Geometry check sheet. Reference: the model listing, model coordinates, mm. A direction names the side the tool comes from. Round coordinates to 2 decimals unless told otherwise and drop trailing zeros. Order: outer loops, then holes, each group sorted by start corner. A loop starts at its lowest first (then second) coordinate and runs counter-clockwise, first axis right, second up. Notation, with made-up numbers: M -6.5,-31 L 47.5,-31 A22 cw 47.5,-4 Z; hole C 79.25,78.5 d3. An arc over 180 degrees is marked long. Answer as a JSON object with one key per item and string values. Group by question number.
```python
from build123d import *

# Parameters (mm, degrees)
BOSS_EXTRUDE1_DEPTH = 2
SKETCH2_R           = 5
BOSS_EXTRUDE3_DEPTH = 4
SKETCH5_R           = 3
CUT_EXTRUDE1_DEPTH  = 4
SKETCH6_R           = 1.5
CUT_EXTRUDE2_DEPTH  = 2
SKETCH7_R           = 2.5
CUT_EXTRUDE4_DEPTH  = 3


with BuildPart() as part:
    # Sketch1 → Boss-Extrude1 (new body)
    with BuildSketch(Plane(origin=(0, 0, 0), x_dir=(1, 0, 0), z_dir=(0, 1, 0))):
        with BuildLine():
            Line((0, 7.598649923), (20, 7.598649923))
            ThreePointArc((20, 7.598649923), (27.5, 0.098649923), (20, -7.401350077))
            Line((20, -7.401350077), (0, -7.401350077))
            ThreePointArc((0, -7.401350077), (-7.5, 0.098649923), (0, 7.598649923))
        make_face()
    extrude(amount=BOSS_EXTRUDE1_DEPTH)

    # Sketch2 → Boss-Extrude3 (add)
    with BuildSketch(Plane(origin=(0, 2, 0), x_dir=(1, 0, 0), z_dir=(0, 1, 0))):
        Circle(SKETCH2_R)
    extrude(amount=BOSS_EXTRUDE3_DEPTH)

    # Sketch5 → Cut-Extrude1 (cut)
    with BuildSketch(Plane(origin=(0, 6, 0), x_dir=(1, 0, 0), z_dir=(0, 1, 0))):
        Circle(SKETCH5_R)
    extrude(amount=-CUT_EXTRUDE1_DEPTH, mode=Mode.SUBTRACT)

    # Sketch6 → Cut-Extrude2 (cut)
    with BuildSketch(Plane(origin=(0, 2, 0), x_dir=(1, 0, 0), z_dir=(0, 1, 0))):
        Circle(SKETCH6_R)
    extrude(amount=-CUT_EXTRUDE2_DEPTH, mode=Mode.SUBTRACT)

    # Sketch7 → Cut-Extrude4 (cut, through all)
    with BuildSketch(Plane(origin=(0, 2, 0), x_dir=(1, 0, 0), z_dir=(0, 1, 0))):
        with Locations((12.2, 0)):
            Circle(SKETCH7_R)
    extrude(amount=-CUT_EXTRUDE4_DEPTH, mode=Mode.SUBTRACT)


solid = part.part
```
1) Sectioned sample at B-B (y = 0.95). Record the boundary of the cut face in (x, z), then the cut area to 3 significant figures.
2) Go/stop test with flat-tipped pins: P1, Ø1.8, axis at x = -1, z = -0.5, coming from the +Y side; P2, Ø1, axis at x = 21, y = 1, coming from the -Z side. Record where each tip stops, or that it passes through.
3) Sectioned sample at D-D (y = 3.75). Record the boundary of the cut face in (x, z), then the cut area to 3 significant figures.
4) Sectioned sample at C-C (z = 1). Record the boundary of the cut face in (x, y), then the cut area to 3 significant figures.
5) Sectioned sample at A-A (x = 12.2). Record the boundary of the cut face in (y, z), then the cut area to 3 significant figures.
6) Thickness scan on line 1 along X through (y, z) = (0.5, 0); line 2 along Z through (x, y) = (12.2, 0.85); line 3 along Y through (x, z) = (24, 1.25). Record the ranges inside material, lowest first. Write a range as [from, to].
7) Release check for a two-part mould opening along X. For faces 1 (the cylindrical face through (-1.08, 3.97, 4.88)), 2 (the cylindrical face through (-3, 4, 0)), 3 (the cylindrical face through (-7.5, 0.99, 0.07)) record: +X half, -X half, draft (parallel to the pull), parting line (faces both ways), or undercut.
8) Set-up check for faces 4 (the cylindrical face through (-1.5, 1.01, -0.07)), 5 (the flat face through (1.3, 2, 1.3)): record each of +Z, -Z, +X, -X, +Y, -Y from which the full face is reachable in a straight line by a thin tool's end or side.
Final values:
{
 "1": {"outline": "M 0,-7.6 L 20,-7.6 A7.5 ccw 20,7.4 L 0,7.4 A7.5 ccw Z; hole C 0,0 d3; hole C 12.2,0 d5", "area": "450 mm^2"},
 "2": {"P1": "stops at y = 2", "P2": "stops at z = -7.58"},
 "3": {"outline": "C 0,0 d10; hole C 0,0 d6", "area": "50.3 mm^2"},
 "4": {"outline": "M -7.42,0 L -1.12,0 L -1.12,2 L -2.83,2 L -2.83,6 L -4.9,6 L -4.9,2 L -7.42,2 Z; M 1.12,0 L 9.91,0 L 9.91,2 L 4.9,2 L 4.9,6 L 2.83,6 L 2.83,2 L 1.12,2 Z; M 14.49,0 L 27.42,0 L 27.42,2 L 14.49,2 Z", "area": "72.6 mm^2"},
 "5": {"outline": "M 0,-7.6 L 2,-7.6 L 2,-2.5 L 0,-2.5 Z; M 0,2.5 L 2,2.5 L 2,7.4 L 0,7.4 Z", "area": "20.0 mm^2"},
 "6": {"line 1": "x = [-7.5, -1.5], [1.5, 9.7], [14.7, 27.5]", "line 2": "z = [-7.6, -2.5], [2.5, 7.4]", "line 3": "y = [0, 2]"},
 "7": {"face 1": "parting line", "face 2": "undercut", "face 3": "-X half"},
 "8": {"face 4": "+Y, -Y", "face 5": "+Y"}
}
